```python
from build123d import *

# Parameters (mm, degrees)
SKETCH1_R           = 2.95
BOSS_EXTRUDE1_DEPTH = 2.5
SKETCH2_R           = 1.5
BOSS_EXTRUDE2_DEPTH = 35
CHAMFER1_SIZE       = 0.3
CUT_EXTRUDE1_DEPTH  = 2
FILLET1_R           = 1


with BuildPart() as part:
    # Sketch1 → Boss-Extrude1 (new body)
    with BuildSketch(Plane.XY):
        Circle(SKETCH1_R)
    extrude(amount=BOSS_EXTRUDE1_DEPTH)

    # Sketch2 → Boss-Extrude2 (add)
    with BuildSketch(Plane(origin=(0, 0, 0), x_dir=(-1, 0, 0), z_dir=(0, 0, -1))):
        with Locations(Location((0, 0, 0), (0, 0, 180))):
            Circle(SKETCH2_R)
    extrude(amount=BOSS_EXTRUDE2_DEPTH)

    # Chamfer1
    chamfer1_edges = [part.edges().sort_by_distance(p)[0] for p in [
        (-1.5, 0, -35),
    ]]
    chamfer(chamfer1_edges, length=CHAMFER1_SIZE)

    # Sketch3 → Cut-Extrude1 (cut)
    with BuildSketch(Plane.XY.offset(2.5)):
        Polygon((0.363589324, 0.363589324), (2, 0.363589324), (2, -0.363589324), (0.363589324, -0.363589324), (0.363589324, -2), (-0.363589324, -2), (-0.363589324, -0.363589324), (-2, -0.363589324), (-2, 0.363589324), (-0.363589324, 0.363589324), (-0.363589324, 2), (0.363589324, 2), align=None)
    extrude(amount=-CUT_EXTRUDE1_DEPTH, mode=Mode.SUBTRACT)

    # Fillet1
    # the kernel refuses this fillet: 1 mm, written as the material it takes off along each edge
    with BuildSketch(Plane(origin=(0, 0, 2.5), x_dir=(1, 0, 0), z_dir=(0, -1, 0))) as fillet1_piece_1:
        with BuildLine():
            CenterArc((2.95 - FILLET1_R, -FILLET1_R), FILLET1_R, 0, 90)
            Line((2.95 - FILLET1_R, 0), (2.95, 0))
            Line((2.95, 0), (2.95, -FILLET1_R))
        make_face()
    revolve(axis=Axis((0, 0, 2.5), (0, 0, 1)), mode=Mode.SUBTRACT)


solid = part.part
```
Source: CAD feature listing. Evaluate the final solid. Frame: model axes, mm. A direction names the side the tool comes from. Give positions to 0.01 mm unless a question says otherwise; leave off trailing zeros. Order: outer loops, then holes, each group sorted by start corner. A loop starts at its lowest first (then second) coordinate and runs counter-clockwise, first axis right, second up.
(1) Contact query for flat-ended pins moving along their axis: P1, Ø1.8, axis at x = -1, z = 1, coming from the +Y side; P2, Ø1, axis at x = 2, y = 1.5, coming from the -Z side; P3, Ø0.8, axis at y = -1.5, z = 1.5, coming from the -X side. Output: stop coordinate, or through.
(2) Pull-direction query (X, two-part tool) for faces 1 (the face through (1.43, -0.45, -17.11)), 2 (the face through (1, -0.364, 2)), 3 (the face through (-1, 1, 2.5)); classes: +X half, -X half, draft (parallel to the pull), parting line (faces both ways), or undercut.
(3) Material intervals for line 1 along Z through (x, y) = (-1.4, -1.5); line 2 along Z through (x, y) = (0.5, -0.1); line 3 along X through (y, z) = (0.1, -22.5), sorted ascending.
(4) Access query for faces 4 (the face through (-1, -1, 2.5)), 5 (the face through (1.3, -1.3, 0)), 6 (the face through (1, 0.364, 2)). Directions: +Z, -Z, +X, -X, +Y, -Y. A direction counts if a zero-diameter tool reaches every point of the face in a straight line with its end or side. Return the directions, or none.
(5) Section query A-A (y = 0). Return the cut outline in (x, z).
(6) Section query B-B (z = -31.5). Return the cut outline in (x, y), plus the area to 3 significant figures.
Outcome:
1. P1: stops at y = 2.95
1. P2: stops at z = 0
1. P3: stops at x = -2.74
2. face 1: parting line
2. face 2: undercut
2. face 3: draft
3. line 1: z = 0 to 2.49
3. line 2: z = -35 to 0.5
3. line 3: x = -1.5 to 1.5
4. face 4: +Z, +X, -X, +Y, -Y
4. face 5: -Z
4. face 6: +Z
5. outline: (-2.95, 0) - (-1.5, 0) - (-1.5, -34.7) - (-1.2, -35) - (1.2, -35) - (1.5, -34.7) - (1.5, 0) - (2.95, 0) - (2.95, 1.5) arc R1 ccw to (2, 2.5) - (2, 0.5) - (-2, 0.5) - (-2, 2.5) arc R1 ccw to (-2.95, 1.5) - close
6. outline: circle Ø3 at (0, 0)
6. area: 7.07 mm2
